Drawing for the job (mm, zero at the part's lowest x, y, z). A direction names the side the tool comes from. Give positions to 0.01 mm unless a question says otherwise; leave off trailing zeros. Order: outer loops, then holes, each group sorted by start corner. A loop starts at its lowest first (then second) coordinate and runs counter-clockwise, first axis right, second up. Notation, with made-up numbers: (-33, -16) - (-20, -16) arc R28 cw to (-20, 3) - close; hole circle Ø5 at (64.5, 18.5). An arc over 180 degrees is marked (long way). Use a Markdown table: item, result. Add a question column.
(1) Slice it at A-A (y = 25.4). Write the cut outline in (x, z).
(2) Mould opens along Y. For the marked faces 4, 5, 6 and 7 say: +Y half, -Y half, draft (parallel to the pull), parting line (faces both ways), or undercut.
(3) Slice it at D-D (y = 45). Write the cut outline in (x, z).
(4) Flat gauge pins, fed straight in: pin 1 (1 mm diameter, centred on y = 36, z = 10, fed in from -X); pin 2 (2 mm diameter, centred on y = 37.5, z = 12, fed in from +X); pin 3 (8 mm diameter, centred on x = 37, y = 9.5, fed in from +Z). Where does each tip first touch, or does it go through?
(5) Slice it at C-C (x = 38.1). Write the cut outline in (y, z), then the cut area to 3 significant figures.
(6) Which spindle directions (+Z, -Z, +X, -X, +Y, -Y) get a long thin tool onto all of the face, cutting with end or side? Do the marked faces 1, 2 and 3. Say none if no direction does.
(7) Slice it at B-B (z = 6.35). Write the cut outline in (x, y).
(8) Wall check: line 1 (Y direction, x = 38.1, z = 8); line 2 (X direction, y = 25.4, z = 8.25) (1 decimal); line 3 (X direction, y = 25.4, z = 6). Give the ranges that are in metal, low to high.
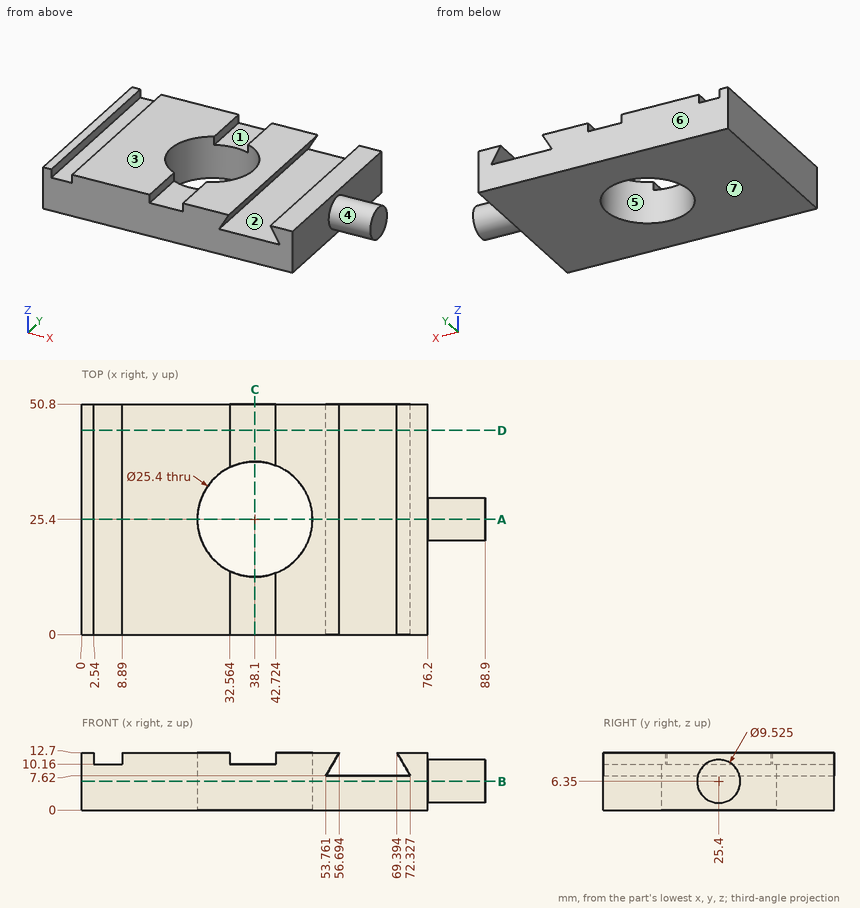
Solution:
| question | item | result |
|---|---|---|
| 1 | outline | (0, 0) - (25.4, 0) - (25.4, 12.7) - (8.89, 12.7) - (8.89, 10.16) - (2.54, 10.16) - (2.54, 12.7) - (0, 12.7) - close; (50.8, 0) - (76.2, 0) - (76.2, 1.59) - (88.9, 1.59) - (88.9, 11.11) - (76.2, 11.11) - (76.2, 12.7) - (69.39, 12.7) - (72.33, 7.62) - (53.76, 7.62) - (56.69, 12.7) - (50.8, 12.7) - close |
| 2 | face 4 | parting line |
| 2 | face 5 | undercut |
| 2 | face 6 | +Y half |
| 2 | face 7 | draft |
| 3 | outline | (0, 0) - (76.2, 0) - (76.2, 12.7) - (69.39, 12.7) - (72.33, 7.62) - (53.76, 7.62) - (56.69, 12.7) - (42.72, 12.7) - (42.72, 10.16) - (32.56, 10.16) - (32.56, 12.7) - (8.89, 12.7) - (8.89, 10.16) - (2.54, 10.16) - (2.54, 12.7) - (0, 12.7) - close |
| 4 | pin 1 | x = 0 |
| 4 | pin 2 | x = 76.2 |
| 4 | pin 3 | z = 10.16 |
| 5 | outline | (0, 0) - (12.7, 0) - (12.7, 10.16) - (0, 10.16) - close; (38.1, 0) - (50.8, 0) - (50.8, 10.16) - (38.1, 10.16) - close |
| 5 | area | 258 mm2 |
| 6 | face 1 | +Z, +Y, -Y |
| 6 | face 2 | +Y, -Y |
| 6 | face 3 | +Z, +X, -X, +Y, -Y |
| 7 | outline | (0, 0) - (76.2, 0) - (76.2, 20.64) - (88.9, 20.64) - (88.9, 30.16) - (76.2, 30.16) - (76.2, 50.8) - (0, 50.8) - close; hole circle Ø25.4 at (38.1, 25.4) |
| 8 | line 1 | 0 to 12.7, 38.1 to 50.8 |
| 8 | line 2 | 0 to 25.4, 50.8 to 54.1, 72 to 88.9 |
| 8 | line 3 | 0 to 25.4, 50.8 to 88.9 |
